```python
from build123d import *

# Parameters (mm, degrees)
BOSS_EXTRUDE1_DEPTH = 6
FILLET1_R           = 10
SKETCH2_R           = 2.5
CUT_EXTRUDE1_DEPTH  = 6
SKETCH5_R           = 7.5
CUT_EXTRUDE3_DEPTH  = 4
SKETCH6_R           = 5.5
CUT_EXTRUDE4_DEPTH  = 4
SKETCH8_W           = 16
SKETCH8_H           = 121.699623713
CUT_EXTRUDE5_DEPTH  = 2
FILLET2_R           = 10
CUT_EXTRUDE6_DEPTH  = 10
SKETCH10_R          = 1.25
CUT_EXTRUDE7_DEPTH  = 10
SKETCH11_R          = 1.25
CUT_EXTRUDE8_DEPTH  = 10
SKETCH12_R          = 1.65
CUT_EXTRUDE9_DEPTH  = 10


with BuildPart() as part:
    # Sketch1 → Boss-Extrude1 (new body)
    with BuildSketch(Plane(origin=(0, 0, 0), x_dir=(1, 0, 0), z_dir=(0, 1, 0))):
        Polygon((21.213083016, -102.227633762), (35.213083016, -90.480238926), (35.213083016, -30.480238926), (21.213083016, -18.73284409), (21.213083016, 31.26715591), (35.213083016, 43.014550747), (35.213083016, 103.014550747), (-36.786916984, 103.014550747), (-36.786916984, 43.014550747), (-22.786916984, 31.26715591), (-22.786916984, -18.73284409), (-36.786916984, -30.480238926), (-36.786916984, -90.480238926), (-22.786916984, -102.227633762), align=None)
    extrude(amount=BOSS_EXTRUDE1_DEPTH)

    # Fillet1
    fillet1_edges = [part.edges().sort_by_distance(p)[0] for p in [
        (-22.786916984, 3, 102.227633762),
        (-36.786916984, 3, 90.480238926),
        (-36.786916984, 3, 30.480238926),
        (-22.786916984, 3, 18.73284409),
        (21.213083016, 3, 18.73284409),
        (35.213083016, 3, 30.480238926),
        (35.213083016, 3, 90.480238926),
        (21.213083016, 3, 102.227633762),
    ]]
    fillet(fillet1_edges, radius=FILLET1_R)

    # Sketch2 → Cut-Extrude1 (cut)
    with BuildSketch(Plane.XZ):
        with Locations(Location((-0.786916984, 60.480238926, 0), (0, 0, 270))):
            Circle(SKETCH2_R)
    extrude(amount=-CUT_EXTRUDE1_DEPTH, mode=Mode.SUBTRACT)

    # Sketch5 → Cut-Extrude3 (cut)
    with BuildSketch(Plane.XZ):
        with Locations(Location((-0.786916984, 60.480238926, 0), (0, 0, 270))):
            Circle(SKETCH5_R)
    extrude(amount=-CUT_EXTRUDE3_DEPTH, mode=Mode.SUBTRACT)

    # Sketch6 → Cut-Extrude4 (cut)
    with BuildSketch(Plane.XZ.offset(-4)):
        with Locations(Location((-0.786916984, 60.480238926, 0), (0, 0, 270))):
            Circle(SKETCH6_R)
    extrude(amount=-CUT_EXTRUDE4_DEPTH, mode=Mode.SUBTRACT)

    # Sketch8 → Cut-Extrude5 (cut)
    with BuildSketch(Plane(origin=(0, 6, 0), x_dir=(1, 0, 0), z_dir=(0, 1, 0))):
        with Locations((-0.786916984, 9.974259286)):
            Rectangle(SKETCH8_W, SKETCH8_H)
    extrude(amount=-CUT_EXTRUDE5_DEPTH, mode=Mode.SUBTRACT)

    # Fillet2
    fillet2_edges = [part.edges().sort_by_distance(p)[0] for p in [
        (-22.786916984, 3, -31.26715591),
        (-36.786916984, 3, -43.014550747),
        (35.213083016, 3, -43.014550747),
        (21.213083016, 3, -31.26715591),
    ]]
    fillet(fillet2_edges, radius=FILLET2_R)

    # Sketch9 → Cut-Extrude6 (cut)
    with BuildSketch(Plane(origin=(0, 6, 0), x_dir=(1, 0, 0), z_dir=(0, 1, 0))):
        with BuildLine():
            Line((7.213083016, 67.824071143), (-8.786916984, 67.824071143))
            ThreePointArc((-8.786916984, 67.824071143), (-11.786916984, 70.824071143), (-8.786916984, 73.824071143))
            Line((-8.786916984, 73.824071143), (7.213083016, 73.824071143))
            ThreePointArc((7.213083016, 73.824071143), (10.213083016, 70.824071143), (7.213083016, 67.824071143))
        make_face()
    extrude(amount=-CUT_EXTRUDE6_DEPTH, mode=Mode.SUBTRACT)

    # Sketch10 → Cut-Extrude7 (cut)
    with BuildSketch(Plane.XZ):
        with Locations(Location((-16.786916984, -6.26715591, 0), (0, 0, 270))):
            Circle(SKETCH10_R)
        with Locations(Location((15.213083016, -6.26715591, 0), (0, 0, 270))):
            Circle(SKETCH10_R)
    extrude(amount=-CUT_EXTRUDE7_DEPTH, mode=Mode.SUBTRACT)

    # Sketch11 → Cut-Extrude8 (cut)
    with BuildSketch(Plane(origin=(0, 6, 0), x_dir=(1, 0, 0), z_dir=(0, 1, 0))):
        with Locations(Location((20.993582106, -90.043344962, 0), (0, 0, 270))):
            Circle(SKETCH11_R)
        with Locations(Location((-22.567416075, -90.043344962, 0), (0, 0, 270))):
            Circle(SKETCH11_R)
    extrude(amount=-CUT_EXTRUDE8_DEPTH, mode=Mode.SUBTRACT)

    # Sketch12 → Cut-Extrude9 (cut)
    with BuildSketch(Plane(origin=(0, 6, 0), x_dir=(1, 0, 0), z_dir=(0, 1, 0))):
        with Locations(Location((25.213083016, 73.014550747, 0), (0, 0, 270))):
            Circle(SKETCH12_R)
        with Locations(Location((-26.786916984, 73.014550747, 0), (0, 0, 270))):
            Circle(SKETCH12_R)
    extrude(amount=-CUT_EXTRUDE9_DEPTH, mode=Mode.SUBTRACT)


solid = part.part
```
Model file for the job. Use its own axes, mm. A direction names the side the tool comes from. Give positions to 0.01 mm unless a question says otherwise; leave off trailing zeros. Order: outer loops, then holes, each group sorted by start corner. A loop starts at its lowest first (then second) coordinate and runs counter-clockwise, first axis right, second up.
1) Saw through at A-A, the plane z = 40.5. Write the cut outline in (x, y).
2) 3-axis set-ups, long thin cutter, end or side, ignore diameter. For faces 4 (the flat face through (-1, 2, -67.824)), 5 (the cylindrical face through (22.12, 3.04, -30.77)), 6 (the cylindrical face through (-0.457, 1.972, 67.973)): which of +Z, -Z, +X, -X, +Y, -Y reach the whole face in a straight line?
3) Mould opens along X. For faces 1 (the flat face through (0, 3, -103.015)), 2 (the cylindrical face through (-23.698, 3.042, -30.775)), 3 (the cylindrical face through (-11.786, 3.042, -70.758)) say: +X half, -X half, draft (parallel to the pull), parting line (faces both ways), or undercut.
4) Wall check: probe 1 along X at (y, z) = (5.7, -51.5); probe 2 along X at (y, z) = (4.3, 10); probe 3 along Z at (x, y) = (-6, 2.7). Give the ranges that are in metal, low to high.
5) Saw through at D-D, the plane y = 1.8. Count the separate pieces of the cut face and the enclosed holes in it, then the cut area to 3 significant figures.
6) Pin check, flat tips, straight feed: pin 1 (1.5 mm diameter, centred on y = 1.5, z = 17.5, fed in from -X); pin 2 (2 mm diameter, centred on y = 5, z = 2.5, fed in from -X); pin 3 (1 mm diameter, centred on y = 4.5, z = 8, fed in from +X). Stop position of each tip, or through.
7) Saw through at C-C, the plane z = -20.5. Write the cut outline in (x, y).
8) Saw through at B-B, the plane x = 1.5. Write the cut outline in (y, z), then the cut area to 3 significant figures.
Computed:
1. outline: (-36.79, 0) - (35.21, 0) - (35.21, 6) - (7.21, 6) - (7.21, 4) - (-8.79, 4) - (-8.79, 6) - (-36.79, 6) - close
2. face 4: +Y, -Y
2. face 5: +X, +Y, -Y
2. face 6: -Y
3. face 1: draft
3. face 2: -X half
3. face 3: undercut
4. probe 1: x = -36.79 to -8.79, 7.21 to 35.21
4. probe 2: x = -22.79 to -8.79, 7.21 to 21.21
4. probe 3: z = -103.01 to -73.82, -67.82 to 55.09, 65.87 to 102.23
5. separate pieces: 1
5. enclosed holes: 8
5. area: 12,500 mm2
6. pin 1: stops at x = -23.7
6. pin 2: stops at x = -22.79
6. pin 3: stops at x = 21.21
7. outline: (-22.79, 0) - (21.21, 0) - (21.21, 6) - (7.21, 6) - (7.21, 4) - (-8.79, 4) - (-8.79, 6) - (-22.79, 6) - close
8. outline: (0, -103.01) - (6, -103.01) - (6, -73.82) - (0, -73.82) - close; (0, -67.82) - (4, -67.82) - (4, 50.88) - (6, 50.88) - (6, 55.48) - (4, 55.48) - (4, 53.34) - (0, 53.34) - close; (0, 67.62) - (4, 67.62) - (4, 65.48) - (6, 65.48) - (6, 102.23) - (0, 102.23) - close
8. area: 881 mm2
